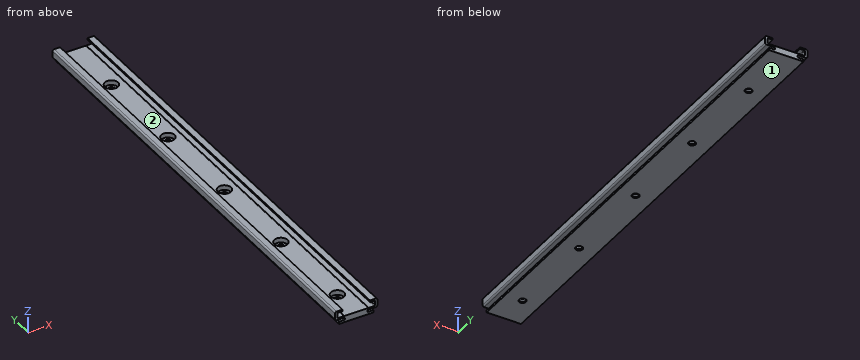
```python
from build123d import *

# Parameters (mm, degrees)
BOSS_EXTRUDE1_DEPTH                              = 300
CUT_EXTRUDE1_DEPTH                               = 301
F_0_4_0_4_DIAMETER_HOLE1_D                       = 0.4
F_0_4_0_4_DIAMETER_HOLE1_DEPTH                   = 300
CBORE_FOR_M4_HEX_HEAD_MACHINE_SCREW1_D           = 4.5
CBORE_FOR_M4_HEX_HEAD_MACHINE_SCREW1_DEPTH       = 4.1
CBORE_FOR_M4_HEX_HEAD_MACHINE_SCREW1_CBORE_D     = 8.5
CBORE_FOR_M4_HEX_HEAD_MACHINE_SCREW1_CBORE_DEPTH = 3.1
FILLET1_R                                        = 0.2
FILLET2_R                                        = 0.5
FILLET3_R                                        = 1


with BuildPart() as part:
    # Sketch1 → Boss-Extrude1 (new body)
    with BuildSketch(Plane(origin=(0, 300, 0), x_dir=(1, 0, 0), z_dir=(0, 1, 0))):
        with BuildLine():
            Line((-13.5, -3), (-13.5, -8.7))
            Line((-13.5, -8.7), (13.5, -8.7))
            Line((13.5, -8.7), (13.5, -3))
            Line((13.5, -3), (7.8, -3))
            ThreePointArc((7.8, -3), (7.05, -2.25), (7.8, -1.5))
            Line((7.8, -1.5), (11, -1.5))
            Line((11, -1.5), (11, 0))
            Line((11, 0), (-11, 0))
            Line((-11, 0), (-11, -1.5))
            Line((-11, -1.5), (-7.8, -1.5))
            ThreePointArc((-7.8, -1.5), (-7.05, -2.25), (-7.8, -3))
            Line((-7.8, -3), (-13.5, -3))
        make_face()
    extrude(amount=-BOSS_EXTRUDE1_DEPTH)

    # Sketch2 → Cut-Extrude1 (cut, through all)
    with BuildSketch(Plane.XZ):
        Polygon((8.75, 8.7), (-8.75, 8.7), (-8.75, 7.6), (-12, 7.6), (-12, 4.1), (12, 4.1), (12, 7.6), (8.75, 7.6), align=None)
    extrude(amount=-CUT_EXTRUDE1_DEPTH, mode=Mode.SUBTRACT)

    # Ø0.4 (0.4) Diameter Hole1
    with Locations(Plane(origin=(0, 300, 0), x_dir=(1, 0, 0), z_dir=(0, 1, 0))):
        with Locations((-7.75, -4.1), (7.75, -4.1)):
            Hole(F_0_4_0_4_DIAMETER_HOLE1_D / 2, depth=F_0_4_0_4_DIAMETER_HOLE1_DEPTH)

    # CBORE for M4 Hex Head Machine Screw1
    with Locations(Plane.XY.offset(4.1)):
        with Locations((0, 260), (0, 200), (0, 140), (0, 80), (0, 20)):
            CounterBoreHole(CBORE_FOR_M4_HEX_HEAD_MACHINE_SCREW1_D / 2, CBORE_FOR_M4_HEX_HEAD_MACHINE_SCREW1_CBORE_D / 2, CBORE_FOR_M4_HEX_HEAD_MACHINE_SCREW1_CBORE_DEPTH, depth=CBORE_FOR_M4_HEX_HEAD_MACHINE_SCREW1_DEPTH)

    # Fillet1
    fillet1_edges = [part.edges().sort_by_distance(p)[0] for p in [
        (-11, 150, 1.5),
        (11, 150, 1.5),
    ]]
    fillet(fillet1_edges, radius=FILLET1_R)

    # Fillet2
    fillet2_edges = [part.edges().sort_by_distance(p)[0] for p in [
        (12, 150, 7.6),
        (12, 150, 4.1),
        (-12, 150, 4.1),
        (-12, 150, 7.6),
    ]]
    fillet(fillet2_edges, radius=FILLET2_R)

    # Fillet3
    fillet3_edges = [part.edges().sort_by_distance(p)[0] for p in [
        (13.5, 150, 3),
        (13.5, 150, 8.7),
        (-13.5, 150, 8.7),
        (-13.5, 150, 3),
    ]]
    fillet(fillet3_edges, radius=FILLET3_R)


solid = part.part
```
For this review, take the finished solid that the model builds, in its own axes (mm). Face numbers are marked on the shaded views. Coordinates: 2 decimals unless noted, no trailing zeros. Answer in a Markdown table with one row per item. Add a question column.
Q1. Draft analysis for pull direction X (two halves, no side actions). For the marked faces 1 and 2, state which applies: +X half, -X half, draft (parallel to the pull), parting line (faces both ways), or undercut.
Q2. For probe 1 along Y at (x, z) = (0, 3.4); probe 2 along Y at (x, z) = (0, 0.55); probe 3 along Z at (x, y) = (-9.75, 164), list the stretches that pass through material, from the lowest coordinate up.
Q3. For P1, Ø4, axis at x = 9, z = 6, coming from the +Y side; P2, Ø12, axis at x = 0, y = 101.5, coming from the +Z side; P3, Ø0.5, axis at y = 106, z = 8.5, coming from the -X side; P4, Ø1.4, axis at y = 118.5, z = 0.5, coming from the -X side, all flat-tipped, find the tip position at first contact; note any pin that passes through.
Answer list:
| question | item | result |
|---|---|---|
| 1 | face 1 | draft |
| 1 | face 2 | undercut |
| 2 | probe 1 | y = 0 to 15.75, 24.25 to 75.75, 84.25 to 135.75, 144.25 to 195.75, 204.25 to 255.75, 264.25 to 300 |
| 2 | probe 2 | y = 0 to 17.75, 22.25 to 77.75, 82.25 to 137.75, 142.25 to 197.75, 202.25 to 257.75, 262.25 to 300 |
| 2 | probe 3 | z = 0 to 1.5, 3 to 4.1, 7.6 to 8.7 |
| 3 | P1 | stops at y = 300 |
| 3 | P2 | stops at z = 4.1 |
| 3 | P3 | stops at x = -13.34 |
| 3 | P4 | stops at x = -11 |
